```python
from build123d import *

# Parameters (mm, degrees)
F1_DEPTH = 7.7
F2_R     = 0.9
F3_DEPTH = 7.7
F4_R     = 5


with BuildPart() as f1:
    # F0 (on Top) → F1 (new body)
    with BuildSketch(Plane.XY):
        Polygon((0, -8), (0, 0), (-8, 0), (-8, 16), (-60.5, 16), (-60.5, -8), align=None)
    extrude(amount=F1_DEPTH)

    # F2 (on face) → F3 (cut, through all)
    with BuildSketch(Plane.XY.offset(7.7)):
        with Locations((-55, 4.5)):
            Circle(F2_R)
        with Locations((-55, -5.5)):
            Circle(F2_R)
        Polygon((-12.75, 8.9), (-8, 8.9), (-8, 12.1), (-12.75, 12.1), (-12.75, 13.4), (-15.25, 13.4), (-15.25, 12.1), (-20, 12.1), (-20, 8.9), (-15.25, 8.9), (-15.25, 7.6), (-12.75, 7.6), align=None)
    extrude(amount=-F3_DEPTH, mode=Mode.SUBTRACT)

    # F4
    f4_edges = [f1.edges().sort_by_distance(p)[0] for p in [
        (-60.5, 16, 3.85),
        (-60.5, -8, 3.85),
    ]]
    fillet(f4_edges, radius=F4_R)


solid = f1.part
```
Verification items for the finished model (mm, model axes). A direction names the side the tool comes from. Give positions to 0.01 mm unless a question says otherwise; leave off trailing zeros. Loops run counter-clockwise (first coordinate to the right, second up) from the corner with the lowest first, then second, coordinate; pieces in that order, holes last.
1. Thickness scan on line 1 (Y direction, x = -55, z = 3.5); line 2 (Y direction, x = -17, z = 5.5); line 3 (Y direction, x = -13, z = 4.5). Record the ranges inside material, lowest first.
2. Go/stop test with flat-tipped pins: pin 1 Ø0.7 at (y, z) = (13, 3) entering from +X; pin 2 Ø4 at (x, z) = (-5.5, 2.5) entering from +Y. Record where each tip stops, or that it passes through.
3. Mould release check, pull along Y, two halves, no side actions. Record for faces 1 (the flat face through (-14, 7.6, 4)), 2 (the cylindrical face through (-59, -6.57, 3.9)), 3 (the flat face through (-31, 4, 7.7)), 4 (the flat face through (-31, 16, 4)): released by +Y, released by -Y, zero draft, split by the parting line, or undercut.
4. Section check A-A, the plane y = 4.5. Enter the section's corners in (x, z), then the cut area to 3 significant figures.
5. Section check B-B, the plane z = 2. Enter the section's corners in (x, y), then the cut area to 3 significant figures.
6. Section check C-C, the plane y = -5.5. Enter the section's corners in (x, z).
7. Set-up check for faces 5 (the flat face through (-60.5, 4, 4)), 6 (the flat face through (-14, 13.4, 4)), 7 (the cylindrical face through (-59.07, 14.5, 3.9)), 8 (the flat face through (-4, 0, 4)), 9 (the flat face through (-20, 11, 4)): record each of +Z, -Z, +X, -X, +Y, -Y from which the full face is reachable in a straight line by a thin tool's end or side.
8. Section check D-D, the plane x = -5. Enter the section's corners in (y, z), then the cut area to 3 significant figures.
Geometry says:
1. line 1: y = -8 to -6.4, -4.6 to 3.6, 5.4 to 16
1. line 2: y = -8 to 8.9, 12.1 to 16
1. line 3: y = -8 to 7.6, 13.4 to 16
2. pin 1: stops at x = -8
2. pin 2: stops at y = 0
3. face 1: undercut
3. face 2: released by -Y
3. face 3: zero draft
3. face 4: released by +Y
4. outline: (-60.5, 0) - (-55.9, 0) - (-55.9, 7.7) - (-60.5, 7.7) - close; (-54.1, 0) - (-8, 0) - (-8, 7.7) - (-54.1, 7.7) - close
4. area: 390 mm2
5. outline: (-60.5, -3) arc R5 ccw to (-55.5, -8) - (0, -8) - (0, 0) - (-8, 0) - (-8, 8.9) - (-12.75, 8.9) - (-12.75, 7.6) - (-15.25, 7.6) - (-15.25, 8.9) - (-20, 8.9) - (-20, 12.1) - (-15.25, 12.1) - (-15.25, 13.4) - (-12.75, 13.4) - (-12.75, 12.1) - (-8, 12.1) - (-8, 16) - (-55.5, 16) arc R5 ccw to (-60.5, 11) - close; hole circle Ø1.8 at (-55, -5.5); hole circle Ø1.8 at (-55, 4.5)
5. area: 1,260 mm2
6. outline: (-59.83, 0) - (-55.9, 0) - (-55.9, 7.7) - (-59.83, 7.7) - close; (-54.1, 0) - (0, 0) - (0, 7.7) - (-54.1, 7.7) - close
7. face 5: +Z, -Z, -X, +Y, -Y
7. face 6: +Z, -Z
7. face 7: +Z, -Z, -X, +Y
7. face 8: +Z, -Z, +X, +Y
7. face 9: +Z, -Z, +X
8. outline: (-8, 0) - (0, 0) - (0, 7.7) - (-8, 7.7) - close
8. area: 61.6 mm2
